```python
from build123d import *

# Parameters (mm, degrees)
F0_W      = 177.8
F0_H      = 76.2
F1_DEPTH  = 76.2
F2_W      = 38.1
F2_H      = 38.1
F3_DEPTH  = 76.2
F4_W      = 25.4
F4_H      = 76.2
F5_DEPTH  = 25.4
F6_W      = 25.4
F6_H      = 76.2
F7_DEPTH  = 15.748
F8_W      = 38.1
F8_H      = 38.1
F10_W     = 38.1
F10_H     = 66.548
F13_DEPTH = 76.2
F15_DEPTH = 101.6
F17_DEPTH = 15.748
F19_DEPTH = 38.1
F20_W     = 12.7
F20_H     = 12.7
F21_DEPTH = 127


with BuildPart() as f1:
    # F0 (on Top) → F1 (new body)
    with BuildSketch(Plane.XY):
        Rectangle(F0_W, F0_H)
    extrude(amount=F1_DEPTH)

    # F2 (on face) → F3 (cut)
    with BuildSketch(Plane.XY.offset(76.2)):
        with Locations((-69.85, -19.05)):
            Rectangle(F2_W, F2_H)
    extrude(amount=-F3_DEPTH, mode=Mode.SUBTRACT)

    # F4 (on face) → F5 (cut)
    with BuildSketch(Plane.XY.offset(76.2)):
        with Locations((76.2, 0)):
            Rectangle(F4_W, F4_H)
    extrude(amount=-F5_DEPTH, mode=Mode.SUBTRACT)

    # F6 (on face) → F7 (join)
    with BuildSketch(Plane(origin=(0, 0, 0), x_dir=(1, 0, 0), z_dir=(0, 0, -1))):
        with Locations((76.2, 0)):
            Rectangle(F6_W, F6_H)
    extrude(amount=F7_DEPTH)

    # F8 (on face) → F9 (revolve)
    with BuildSketch(Plane(origin=(-88.9, 0, 0), x_dir=(0, -1, 0), z_dir=(-1, 0, 0))):
        with Locations((-19.05, 57.15)):
            Rectangle(F8_W, F8_H)
    revolve(axis=Axis((-88.9, 19.05, 38.1), (0, -1, 0)))

    # F10 (on face) → F11 (revolve)
    with BuildSketch(Plane.YZ.offset(88.9)):
        with Locations((19.05, 17.526)):
            Rectangle(F10_W, F10_H)
    revolve(axis=Axis((88.9, 0, 17.526), (0, 0, -1)))

    # F12 (on face) → F13 (cut)
    with BuildSketch(Plane.XZ.offset(38.1)):
        Polygon((48.835303, 76.2), (63.5, 50.8), (63.5, 76.2), align=None)
    extrude(amount=-F13_DEPTH, mode=Mode.SUBTRACT)

    # F14 (on face) → F15 (cut)
    with BuildSketch(Plane.XY.offset(50.8)):
        with BuildLine():
            ThreePointArc((76.2, 0), (79.919744, -8.980256), (88.9, -12.7))
            Line((88.9, -12.7), (88.9, 0))
            Line((88.9, 0), (76.2, 0))
        make_face()
        with BuildLine():
            Line((88.9, 0), (88.9, -12.7))
            ThreePointArc((88.9, -12.7), (97.880256, -8.980256), (101.6, 0))
            ThreePointArc((101.6, 0), (88.9, 12.7), (76.2, 0))
            Line((76.2, 0), (88.9, 0))
        make_face()
    extrude(amount=-F15_DEPTH, mode=Mode.SUBTRACT)

    # F16 (on face) → F17 (cut)
    with BuildSketch(Plane(origin=(0, 0, -15.748), x_dir=(1, 0, 0), z_dir=(0, 0, -1))):
        with BuildLine():
            Line((63.5, -28.398063), (63.5, 28.398063))
            ThreePointArc((63.5, 28.398063), (50.8, 0), (63.5, -28.398063))
        make_face()
    extrude(amount=-F17_DEPTH, mode=Mode.SUBTRACT)

    # F18 (on face) → F19 (cut)
    with BuildSketch(Plane.XZ):
        with BuildLine():
            ThreePointArc((-76.2, 38.1), (-79.919744, 47.080256), (-88.9, 50.8))
            Line((-88.9, 50.8), (-88.9, 38.1))
            Line((-88.9, 38.1), (-76.2, 38.1))
        make_face()
        with BuildLine():
            Line((-88.9, 38.1), (-88.9, 50.8))
            ThreePointArc((-88.9, 50.8), (-97.880256, 29.119744), (-76.2, 38.1))
            Line((-76.2, 38.1), (-88.9, 38.1))
        make_face()
    extrude(amount=-F19_DEPTH, mode=Mode.SUBTRACT)

    # F20 (on face) → F21 (cut)
    with BuildSketch(Plane(origin=(-50.8, 0, 0), x_dir=(0, -1, 0), z_dir=(-1, 0, 0))):
        with Locations((31.75, 69.85)):
            Rectangle(F20_W, F20_H)
    extrude(amount=-F21_DEPTH, mode=Mode.SUBTRACT)


solid = f1.part
```
Build history of the part. All positions in model axes, mm. A direction names the side the tool comes from. Coordinates: 2 decimals unless noted, no trailing zeros. Order: outer loops, then holes, each group sorted by start corner. A loop starts at its lowest first (then second) coordinate and runs counter-clockwise, first axis right, second up.
Item 1: Saw through at A-A on y = -7. List the corners of the cut face in (x, z).
Filled in:
outline: (-50.8, 0) - (63.5, 0) - (63.5, -15.75) - (78.3, -15.75) - (78.3, 50.8) - (63.5, 50.8) - (48.84, 76.2) - (-50.8, 76.2) - close; (99.5, -15.75) - (126.35, -15.75) - (126.35, 50.8) - (99.5, 50.8) - close
Item 2: Saw through at B-B on x = 95.5. List the corners of the cut face in (y, z), then the cut area to 3 significant figures.
Filled in:
outline: (-37.52, -15.75) - (-10.85, -15.75) - (-10.85, 50.8) - (-37.52, 50.8) - close; (10.85, -15.75) - (37.52, -15.75) - (37.52, 50.8) - (10.85, 50.8) - close
area: 3,550 mm2
Item 3: Saw through at C-C on y = 18. List the corners of the cut face in (x, z).
Filled in:
outline: (-88.9, 0) - (63.5, 0) - (63.5, -15.75) - (122.48, -15.75) - (122.48, 50.8) - (63.5, 50.8) - (48.84, 76.2) - (-88.9, 76.2) arc R38.1 ccw to start; hole circle Ø25.4 at (-88.9, 38.1)
Item 4: Drill centre lines: L1, parallel to Z at x = -88.9, y = 28; L2, parallel to Y at x = -67.5, z = 65.5; L3, parallel to X at y = 18, z = 38. Where is each one in solid material? Low to high.
Filled in:
L1: z = 0 to 25.4, 50.8 to 76.2
L2: y = 0 to 38.1
L3: x = -127 to -101.6, -76.2 to 122.48
Item 5: Drop flat-ended pins along their axis: pin 1 Ø4 at (x, y) = (-61.5, 11.5) entering from -Z; pin 2 Ø1.5 at (x, y) = (58.5, 19) entering from +Z; pin 3 Ø10 at (x, z) = (-10.5, 70) entering from -Y. Give the stop position or say it passes through.
Filled in:
pin 1: stops at z = 0
pin 2: stops at z = 60.76
pin 3: stops at y = -25.4
Item 6: Tool access for faces 1 (the flat face through (102, 1, 50.8)), 2 (the flat face through (-73, 0, 39)), 3 (the flat face through (2, -25.4, 70)), 4 (the flat face through (-14, 1, 0)): list every direction of +Z, -Z, +X, -X, +Y, -Y with a clear straight run to the whole face (end or side of a thin tool).
Filled in:
face 1: +Z, +X, +Y, -Y
face 2: +Z, -Z, -X, -Y
face 3: +Z, +X, -X, -Y
face 4: -Z, -X, +Y, -Y
Item 7: Saw through at D-D on z = 55. List the corners of the cut face in (x, y), then the cut area to 3 significant figures.
Filled in:
outline: (-123.05, 0) - (-50.8, 0) - (-50.8, -38.1) - (61.08, -38.1) - (61.08, 38.1) - (-123.05, 38.1) - close
area: 11,300 mm2
